from build123d import *

# Parameters (mm, degrees)
F0_W     = 100
F0_H     = 100
F1_DEPTH = 50
F2_W     = 60
F2_H     = 50
F2_R     = 10
F3_DEPTH = 20
F4_R     = 15
F5_DEPTH = 25


with BuildPart() as f1:
    # F0 (on Top) → F1 (new body)
    with BuildSketch(Plane.XY):
        Rectangle(F0_W, F0_H)
    extrude(amount=F1_DEPTH)

    # F2 (on face) → F3 (cut)
    with BuildSketch(Plane.XY.offset(50)):
        with Locations((0, -25)):
            Rectangle(F2_W, F2_H)
        with Locations((-25, 32.067757)):
            Circle(F2_R)
        with Locations((25, 32.067757)):
            Circle(F2_R)
    extrude(amount=-F3_DEPTH, mode=Mode.SUBTRACT)

    # F4 (on face) → F5 (join)
    with BuildSketch(Plane.XY.offset(30)):
        with Locations((0, -25)):
            Circle(F4_R)
    extrude(amount=F5_DEPTH)


solid = f1.part
The listing builds one solid part. Answer for the finished solid, in the listing's coordinates (mm). A direction names the side the tool comes from. Give positions to 0.01 mm unless a question says otherwise; leave off trailing zeros. Write each loop counter-clockwise with the first axis right and the second up, starting at its lowest first coordinate (ties: lowest second). Pieces come first, ordered by that corner, then holes. Notation, with made-up numbers: (-6.75, 57) -> (45.25, 57) arc R23 cw to (45.25, 78) -> close; hole circle Ø9 at (-20, 35.5). An arc over 180 degrees is marked (long way). One line per question, with ' | ' between items. Start each with the question number.
1. Section C-C (x = 25) is taken. Determine the outline of the cut face in (y, z).
2. Section D-D (y = -37) is taken. Determine the outline of the cut face in (x, z).
3. Given pin 1 Ø3 at (x, y) = (37, 38.5) entering from +Z; pin 2 Ø16 at (x, y) = (24, 33) entering from +Z, each flat-ended and moving along its own axis, determine where each tip first touches the part or whether it passes through.
4. Section B-B (y = -25) is taken. Determine the outline of the cut face in (x, z), plus the area to 3 significant figures.
5. Find the intervals of material crossed by probe 1 along Y at (x, z) = (-25, 45.25); probe 2 along X at (y, z) = (26.5, 39.5); probe 3 along X at (y, z) = (-23, 48.5), in increasing order.
6. For faces 1 (the flat face through (0, -25, 55)), 2 (the flat face through (30, -25, 40)), 3 (the flat face through (0, 0, 40)), determine the directions among +Z, -Z, +X, -X, +Y, -Y from which every point of the face is accessible in a straight line to the end or side of a thin tool.
7. For a pull along Y with two mould halves and no side action, classify faces 4 (the cylindrical face through (-19.624, 40.5, 40.14)), 5 (the flat face through (-1, 12, 50)), 6 (the flat face through (-1, 50, 25)) as pulls with the +Y half, pulls with the -Y half, needs draft (parallel to the pull), parting line crosses it, or undercut.
8. Section A-A (x = 0) is taken. Determine the outline of the cut face in (y, z).
Response values:
1) outline: (-50, 0) -> (50, 0) -> (50, 50) -> (42.07, 50) -> (42.07, 30) -> (22.07, 30) -> (22.07, 50) -> (0, 50) -> (0, 30) -> (-50, 30) -> close
2) outline: (-50, 0) -> (50, 0) -> (50, 50) -> (30, 50) -> (30, 30) -> (9, 30) -> (9, 55) -> (-9, 55) -> (-9, 30) -> (-30, 30) -> (-30, 50) -> (-50, 50) -> close
3) pin 1: z = 50 | pin 2: z = 30
4) outline: (-50, 0) -> (50, 0) -> (50, 50) -> (30, 50) -> (30, 30) -> (15, 30) -> (15, 55) -> (-15, 55) -> (-15, 30) -> (-30, 30) -> (-30, 50) -> (-50, 50) -> close | area: 4,550 mm2
5) probe 1: 0 to 22.07, 42.07 to 50 | probe 2: -50 to -33.31, -16.69 to 16.69, 33.31 to 50 | probe 3: -50 to -30, -14.87 to 14.87, 30 to 50
6) face 1: +Z, +X, -X, +Y, -Y | face 2: +Z, -Y | face 3: +Z
7) face 4: undercut | face 5: needs draft | face 6: pulls with the +Y half
8) outline: (-50, 0) -> (50, 0) -> (50, 50) -> (0, 50) -> (0, 30) -> (-10, 30) -> (-10, 55) -> (-40, 55) -> (-40, 30) -> (-50, 30) -> close
